Check sheet for the drawn part. Datum: minimum x, y, z corner. Units: mm. Give positions to 0.01 mm unless a question says otherwise; leave off trailing zeros. Order: outer loops, then holes, each group sorted by start corner. A loop starts at its lowest first (then second) coordinate and runs counter-clockwise, first axis right, second up. Notation, with made-up numbers: M 38,-36 L 92,-36 A11 cw 92,-18 Z; hole C -39,75.5 d2. An arc over 180 degrees is marked long. Answer as CSV lines item,"result". Start each with the question number.
Q1. Section check A-A, the plane z = 77. Record the boundary of the cut face in (x, y).
Q2. Thickness scan on line 1 (Y direction, x = 5, z = 83.5); line 2 (X direction, y = 5.25, z = 48.5). Record the ranges inside material, lowest first.
Q3. Section check C-C, the plane x = 0.75. Record the boundary of the cut face in (y, z), then the cut area to 3 significant figures.
Q4. Go/stop test with flat-tipped pins: pin 1 (3.5 mm diameter, centred on x = 5, y = 5, fed in from +Z); pin 2 (5 mm diameter, centred on x = 2, z = 76.5, fed in from +Y); pin 3 (3 mm diameter, centred on y = 8.5, z = 36.5, fed in from +X). Record where each tip stops, or that it passes through.
Q5. Section check B-B, the plane y = 8. Record the boundary of the cut face in (x, z).
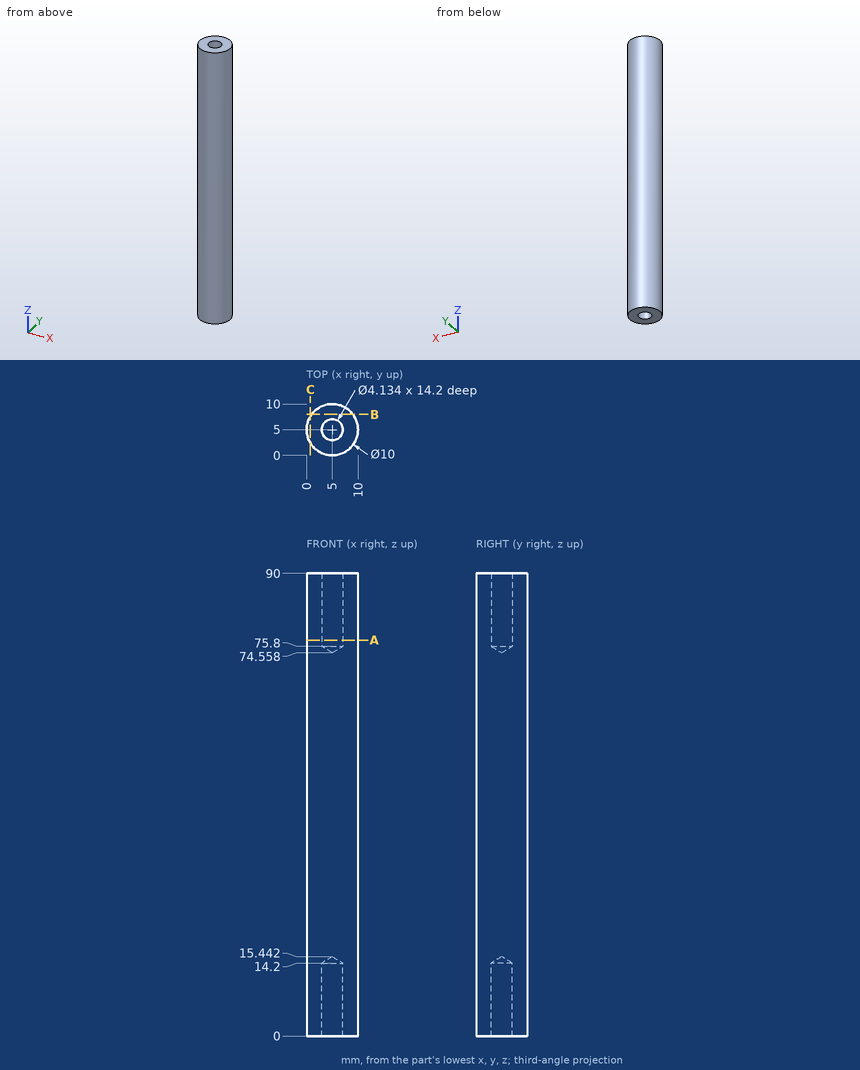
Answer block:
1,outline,"C 5,5 d10; hole C 5,5 d4.13"
2,line 1,"y = 0 to 2.93, 7.07 to 10"
2,line 2,"x = 0.01 to 9.99"
3,outline,"M 2.37,0 L 7.63,0 L 7.63,90 L 2.37,90 Z"
3,area,"474 mm2"
4,pin 1,"stops at z = 75.61"
4,pin 2,"stops at y = 9.97"
4,pin 3,"stops at x = 9.58"
5,outline,"M 1,0 L 9,0 L 9,90 L 1,90 Z"
